Input: part model. Units: mm. Frame: model coordinates. Face numbers are marked on the shaded views. Give positions to 0.01 mm unless a question says otherwise; leave off trailing zeros. Order: outer loops, then holes, each group sorted by start corner. A loop starts at its lowest first (then second) coordinate and runs counter-clockwise, first axis right, second up. Notation, with made-up numbers: (32.5, -5) - (87.5, -5) arc R12 ccw to (87.5, 15) - close; hole circle Ø4 at (-31.75, 54). An arc over 180 degrees is marked (long way). Answer in a Markdown table with one row per item. Add a question column.
1. Mould query, pull axis Y, two halves, no side actions, for the marked faces 1, 2 and 3. Classes: released by +Y, released by -Y, zero draft, split by the parting line, or undercut.
2. Ray query, line 1 (Y direction, x = -12, z = -7); line 2 (Z direction, x = 16.5, y = -3.5); line 3 (X direction, y = -5, z = -6.25). Return the intervals inside material, ascending. Write a range as [from, to].
3. Contact query for flat-ended pins moving along their axis: pin 1 (5.5 mm diameter, centred on x = 12, y = -2.5, fed in from +Z); pin 2 (3.5 mm diameter, centred on x = 12, y = -5, fed in from +Z). Output: stop coordinate, or through.
4. Section query B-B on y = -5. Return loops of the section in (x, z).
5. Section query D-D on z = 0. Return loops of the section in (x, y).
6. Section query C-C on z = -4.5. Return loops of the section in (x, y).
7. Section query A-A on x = -12. Return loops of the section in (y, z).
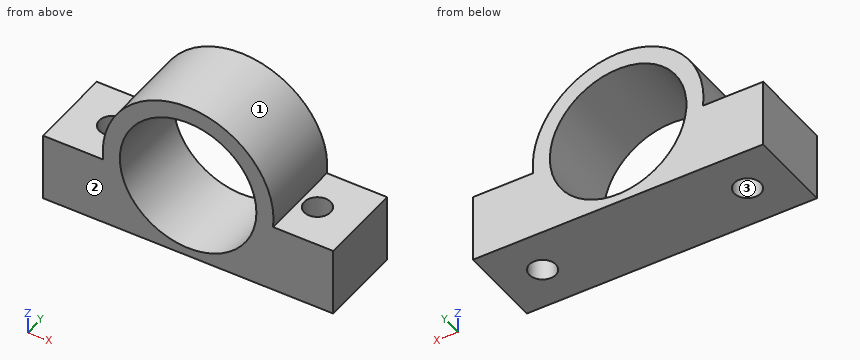
```python
from build123d import *

# Parameters (mm, degrees)
F0_R     = 8
F1_DEPTH = 10
F2_R     = 1.55
F3_DEPTH = 8


with BuildPart() as f1:
    # F0 (on Front) → F1 (new body)
    with BuildSketch(Plane.XZ):
        with BuildLine():
            Line((-17, -1), (-17, -9))
            Line((-17, -9), (17, -9))
            Line((17, -9), (17, -1))
            Line((17, -1), (9.949874, -1))
            ThreePointArc((9.949874, -1), (0, 10), (-9.949874, -1))
            Line((-9.949874, -1), (-17, -1))
        make_face()
        Circle(F0_R, mode=Mode.SUBTRACT)
    extrude(amount=F1_DEPTH)

    # F2 (on face) → F3 (cut, through all)
    with BuildSketch(Plane(origin=(0, 0, -9), x_dir=(1, 0, 0), z_dir=(0, 0, -1))):
        with Locations((-12, 5)):
            Circle(F2_R)
        with Locations((12, 5)):
            Circle(F2_R)
    extrude(amount=-F3_DEPTH, mode=Mode.SUBTRACT)


solid = f1.part
```
Answer:
| question | item | result |
|---|---|---|
| 1 | face 1 | zero draft |
| 1 | face 2 | released by -Y |
| 1 | face 3 | undercut |
| 2 | line 1 | y = [-10, -6.55], [-3.45, 0] |
| 2 | line 2 | z = [-9, -1] |
| 2 | line 3 | x = [-17, -13.55], [-10.45, -4.99], [4.99, 10.45], [13.55, 17] |
| 3 | pin 1 | stops at z = 3.8 |
| 3 | pin 2 | stops at z = -1 |
| 4 | outline | (-17, -9) - (-13.55, -9) - (-13.55, -1) - (-17, -1) - close; (-10.45, -9) - (10.45, -9) - (10.45, -1) - (9.95, -1) arc R10 ccw (long way) to (-9.95, -1) - (-10.45, -1) - close; (13.55, -9) - (17, -9) - (17, -1) - (13.55, -1) - close; hole circle Ø16 at (0, 0) |
| 5 | outline | (-10, -10) - (-8, -10) - (-8, 0) - (-10, 0) - close; (8, -10) - (10, -10) - (10, 0) - (8, 0) - close |
| 6 | outline | (-17, -10) - (-6.61, -10) - (-6.61, 0) - (-17, 0) - close; (6.61, -10) - (17, -10) - (17, 0) - (6.61, 0) - close; hole circle Ø3.1 at (-12, -5); hole circle Ø3.1 at (12, -5) |
| 7 | outline | (-10, -9) - (-6.55, -9) - (-6.55, -1) - (-10, -1) - close; (-3.45, -9) - (0, -9) - (0, -1) - (-3.45, -1) - close |
